Here's the drawing with two shaded views (mm, measured from the low corner). I have some questions. A direction names the side the tool comes from. Round coordinates to 2 decimals unless told otherwise and drop trailing zeros. Loops run counter-clockwise (first coordinate to the right, second up) from the corner with the lowest first, then second, coordinate; pieces in that order, holes last. Notation, with made-up numbers: M -39,29.5 L -3,29.5 A26 cw -3,64.5 Z; hole C -10,14.5 d5. An arc over 180 degrees is marked long. Answer as CSV lines item,"result".
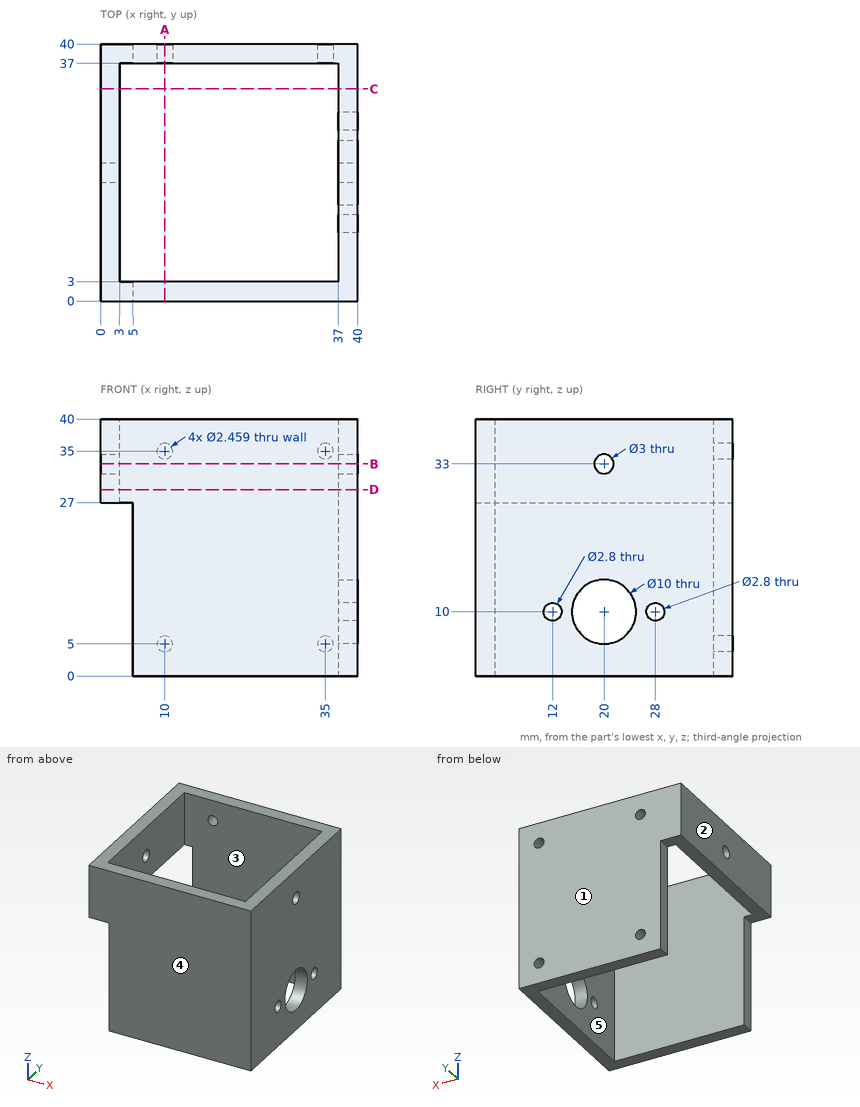
1. I want a section at D-D, the plane z = 29. Please give me the cut outline in (x, y).
Evaluation:
outline,"M 0,0 L 40,0 L 40,40 L 0,40 Z; hole M 3,3 L 37,3 L 37,37 L 3,37 Z"
2. For P1, Ø5.5, axis at x = 3.5, y = 20, coming from the -Z side; P2, Ø11.5, axis at y = 20, z = 10, coming from the -X side; P3, Ø1, axis at y = 18.5, z = 6, coming from the -X side; P4, Ø2, axis at x = 10, z = 35, coming from the +Y side, each with a flat end and sliding along its axis, tell me the tip position at first contact or that it passes through.
Evaluation:
P1,"stops at z = 27"
P2,"stops at x = 37"
P3,"passes through"
P4,"stops at y = 3"
3. I want a section at C-C, the plane y = 33. Please give me the cut outline in (x, z), and give its area (3 significant figures).
Evaluation:
outline,"M 0,27 L 3,27 L 3,40 L 0,40 Z; M 37,0 L 40,0 L 40,40 L 37,40 Z"
area,"159 mm²"
4. We'd pull the mould along Y, two halves only. Please class the marked faces 1, 2 and 3: pulls with the +Y half, pulls with the -Y half, needs draft (parallel to the pull), parting line crosses it, or undercut.
Evaluation:
face 1,"pulls with the +Y half"
face 2,"needs draft"
face 3,"undercut"
5. Which directions (+Z, -Z, +X, -X, +Y, -Y) give clear straight access to the entire face, cutting with the end or side of a thin tool? Please do the marked faces 4 and 5.
Evaluation:
face 4,"+Z, -Z, +X, -X, -Y"
face 5,"+Z, -Z"
6. I want a section at A-A, the plane x = 10. Please give me the cut outline in (y, z), and give its area (3 significant figures).
Evaluation:
outline,"M 0,0 L 3,0 L 3,40 L 0,40 Z; M 37,0 L 40,0 L 40,3.77 L 37,3.77 Z; M 37,6.23 L 40,6.23 L 40,33.77 L 37,33.77 Z; M 37,36.23 L 40,36.23 L 40,40 L 37,40 Z"
area,"225 mm²"
7. If I drill on line 1 (X direction, y = 39.1, z = 5); line 2 (Y direction, x = 39.3, z = 10); line 3 (Y direction, x = 33, z = 10), over which ranges is the centre line in solid material (lowest first)? Write a range as [from, to].
Evaluation:
line 1,"x = [5, 8.77], [11.23, 33.77], [36.23, 40]"
line 2,"y = [0, 10.6], [13.4, 15], [25, 26.6], [29.4, 40]"
line 3,"y = [0, 3], [37, 40]"
8. I want a section at B-B, the plane z = 33. Please give me the cut outline in (x, y), and give its area (3 significant figures).
Evaluation:
outline,"M 0,0 L 40,0 L 40,18.5 L 37,18.5 L 37,3 L 3,3 L 3,18.5 L 0,18.5 Z; M 0,21.5 L 3,21.5 L 3,37 L 37,37 L 37,21.5 L 40,21.5 L 40,40 L 0,40 Z"
area,"426 mm²"
